Verification items for the finished model (mm, model axes). Give positions to 0.01 mm unless a question says otherwise; leave off trailing zeros. Order: outer loops, then holes, each group sorted by start corner. A loop starts at its lowest first (then second) coordinate and runs counter-clockwise, first axis right, second up.
from build123d import *

# Parameters (mm, degrees)
F0_W        = 3.1758
F0_H        = 3.1
F0_W_2      = 1.1684
F0_W_3      = 6.5286
F0_W_4      = 0.9144
F0_W_5      = 6.5226
F0_W_6      = 0.6604
F0_W_7      = 6.5339
F0_W_8      = 0.4318
F0_W_9      = 6.529
F0_W_10     = 0.3302
F0_W_11     = 6.5279
F0_W_12     = 0.254
F0_W_13     = 3.173
F1_DEPTH    = 4
F2_W        = 0.5842
F2_H        = 3.1
F2_W_2      = 0.4572
F2_W_3      = 0.3302
F2_W_4      = 0.2159
F2_W_5      = 0.1651
F2_W_6      = 0.127
F3_DEPTH    = 1.2
F4_T1_DEPTH = 3.1
F5_R        = 0.125
F6_R        = 1.5
F7_R        = 0.2


# Not quite as in the source:
# - a fillet or chamfer that OpenCascade refuses, or shapes differently, is made with other operations: its cross-section is extruded or revolved along the edge and cut away or added


with BuildPart() as f1:
    # F0 (on Top) → F1 (new body)
    with BuildSketch(Plane.XY):
        with Locations((-11.6114438434, -2.5640697926)):
            Rectangle(F0_W, F0_H)
        with Locations((-9.4393438434, -2.5640697926)):
            Rectangle(F0_W_2, F0_H)
        with Locations((-5.5908438434, -2.5640697926)):
            Rectangle(F0_W_3, F0_H)
        with Locations((-1.8693438434, -2.5640697926)):
            Rectangle(F0_W_4, F0_H)
        with Locations((1.8491561566, -2.5640697926)):
            Rectangle(F0_W_5, F0_H)
        with Locations((5.4406561566, -2.5640697926)):
            Rectangle(F0_W_6, F0_H)
        with Locations((9.0378061566, -2.5640697926)):
            Rectangle(F0_W_7, F0_H)
        with Locations((12.5206561566, -2.5640697926)):
            Rectangle(F0_W_8, F0_H)
        with Locations((16.0010561566, -2.5640697926)):
            Rectangle(F0_W_9, F0_H)
        with Locations((19.4306561566, -2.5640697926)):
            Rectangle(F0_W_10, F0_H)
        with Locations((22.8597061566, -2.5640697926)):
            Rectangle(F0_W_11, F0_H)
        with Locations((26.2506561566, -2.5640697926)):
            Rectangle(F0_W_12, F0_H)
        with Locations((27.9641561566, -2.5640697926)):
            Rectangle(F0_W_13, F0_H)
    extrude(amount=F1_DEPTH)

    # F2 (on face) → F3 (cut)
    with BuildSketch(Plane.XY.offset(4)):
        with Locations((-9.1472438434, -2.5640697926)):
            Rectangle(F2_W, F2_H)
        with Locations((-9.7314438434, -2.5640697926)):
            Rectangle(F2_W, F2_H)
        with Locations((-1.6407438434, -2.5640697926)):
            Rectangle(F2_W_2, F2_H)
        with Locations((-2.0979438434, -2.5640697926)):
            Rectangle(F2_W_2, F2_H)
        with Locations((5.2755561566, -2.5640697926)):
            Rectangle(F2_W_3, F2_H)
        with Locations((5.6057561566, -2.5640697926)):
            Rectangle(F2_W_3, F2_H)
        with Locations((12.4127061566, -2.5640697926)):
            Rectangle(F2_W_4, F2_H)
        with Locations((12.6286061566, -2.5640697926)):
            Rectangle(F2_W_4, F2_H)
        with Locations((19.3481061566, -2.5640697926)):
            Rectangle(F2_W_5, F2_H)
        with Locations((19.5132061566, -2.5640697926)):
            Rectangle(F2_W_5, F2_H)
        with Locations((26.3141561566, -2.5640697926)):
            Rectangle(F2_W_6, F2_H)
        with Locations((26.1871561566, -2.5640697926)):
            Rectangle(F2_W_6, F2_H)
    extrude(amount=-F3_DEPTH, mode=Mode.SUBTRACT)

    # F4: fillet of radius 0.25 on 8 edges, made by hand

    # F4_s2 → F4_t1 (join)
    with BuildSketch(Plane.XZ.offset(1.0140697926)):
        with BuildLine():
            ThreePointArc((-10.0235438434, 3.05), (-9.9503205387, 2.8732233047), (-9.7735438434, 2.8))
            Line((-9.7735438434, 2.8), (-10.0235438434, 2.8))
            Line((-10.0235438434, 2.8), (-10.0235438434, 3.05))
        make_face()
        with BuildLine():
            ThreePointArc((-9.1051438434, 2.8), (-8.9283671481, 2.8732233047), (-8.8551438434, 3.05))
            Line((-8.8551438434, 3.05), (-8.8551438434, 2.8))
            Line((-8.8551438434, 2.8), (-9.1051438434, 2.8))
        make_face()
        with BuildLine():
            ThreePointArc((-1.6621438434, 2.8), (-1.4853671481, 2.8732233047), (-1.4121438434, 3.05))
            Line((-1.4121438434, 3.05), (-1.4121438434, 2.8))
            Line((-1.4121438434, 2.8), (-1.6621438434, 2.8))
        make_face()
        with BuildLine():
            ThreePointArc((-2.3265438434, 3.05), (-2.2533205387, 2.8732233047), (-2.0765438434, 2.8))
            Line((-2.0765438434, 2.8), (-2.3265438434, 2.8))
            Line((-2.3265438434, 2.8), (-2.3265438434, 3.05))
        make_face()
        with BuildLine():
            ThreePointArc((5.1104561566, 3.05), (5.1836794613, 2.8732233047), (5.3604561566, 2.8))
            Line((5.3604561566, 2.8), (5.1104561566, 2.8))
            Line((5.1104561566, 2.8), (5.1104561566, 3.05))
        make_face()
        with BuildLine():
            ThreePointArc((5.5208561566, 2.8), (5.6976328519, 2.8732233047), (5.7708561566, 3.05))
            Line((5.7708561566, 3.05), (5.7708561566, 2.8))
            Line((5.7708561566, 2.8), (5.5208561566, 2.8))
        make_face()
        with BuildLine():
            ThreePointArc((12.4865561566, 2.8), (12.6633328519, 2.8732233047), (12.7365561566, 3.05))
            Line((12.7365561566, 3.05), (12.7365561566, 2.8))
            Line((12.7365561566, 2.8), (12.4865561566, 2.8))
        make_face()
        with BuildLine():
            ThreePointArc((12.3047561566, 3.05), (12.3779794613, 2.8732233047), (12.5547561566, 2.8))
            Line((12.5547561566, 2.8), (12.3047561566, 2.8))
            Line((12.3047561566, 2.8), (12.3047561566, 3.05))
        make_face()
    extrude(amount=F4_T1_DEPTH)

    # F5
    f5_edges = [f1.edges().sort_by_distance(p)[0] for p in [
        (19.265556, -2.56407, 2.8),
        (19.595756, -2.56407, 2.8),
        (26.377656, -2.56407, 2.8),
        (26.123656, -2.56407, 2.8),
    ]]
    fillet(f5_edges, radius=F5_R)

    # F6
    f6_edges = [f1.edges().sort_by_distance(p)[0] for p in [
        (29.550656, -2.56407, 4),
        (-13.199344, -2.56407, 4),
    ]]
    fillet(f6_edges, radius=F6_R)

    # F7
    f7_edges = [f1.edges().sort_by_distance(p)[0] for p in [
        (-10.023544, -2.56407, 4),
        (-8.855144, -2.56407, 4),
        (-2.326544, -2.56407, 4),
        (-1.412144, -2.56407, 4),
        (5.110456, -2.56407, 4),
        (5.770856, -2.56407, 4),
        (12.304756, -2.56407, 4),
        (12.736556, -2.56407, 4),
        (19.265556, -2.56407, 4),
        (19.595756, -2.56407, 4),
        (26.123656, -2.56407, 4),
        (26.377656, -2.56407, 4),
    ]]
    fillet(f7_edges, radius=F7_R)


solid = f1.part
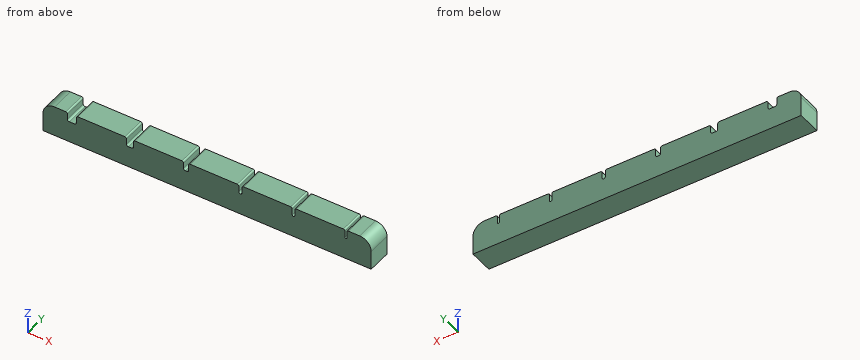
(1) Section check A-A, the plane z = 3.4. Enter the section's corners in (x, y), then the cut area to 3 significant figures.
Solved:
outline: (-12.9, -4.11) - (-10.02, -4.11) - (-10.02, -1.01) - (-12.9, -1.01) - close; (-8.86, -4.11) - (-2.33, -4.11) - (-2.33, -1.01) - (-8.86, -1.01) - close; (-1.41, -4.11) - (5.11, -4.11) - (5.11, -1.01) - (-1.41, -1.01) - close; (5.77, -4.11) - (12.3, -4.11) - (12.3, -1.01) - (5.77, -1.01) - close; (12.74, -4.11) - (19.27, -4.11) - (19.27, -1.01) - (12.74, -1.01) - close; (19.6, -4.11) - (26.12, -4.11) - (26.12, -1.01) - (19.6, -1.01) - close; (26.38, -4.11) - (29.25, -4.11) - (29.25, -1.01) - (26.38, -1.01) - close
area: 119 mm2
(2) Go/stop test with flat-tipped pins: pin 1 (1 mm diameter, centred on y = -3, z = 3.5, fed in from -X); pin 2 (0.6 mm diameter, centred on y = -3, z = 3.5, fed in from +X); pin 3 (1 mm diameter, centred on y = -2, z = 3.5, fed in from +X); pin 4 (1.5 mm diameter, centred on y = -3, z = 3, fed in from +X). Record where each tip stops, or that it passes through.
Solved:
pin 1: stops at x = -13.11
pin 2: stops at x = 29.38
pin 3: stops at x = 29.46
pin 4: stops at x = 29.55
(3) Scan line: line 1 (Z direction, x = -9.5, y = -1.75). Record every from-to range of solid material in increasing order.
Solved:
line 1: z = 0 to 2.8
